Can you work these out from the model? Positions are in its coordinate system, mm. A direction names the side the tool comes from. Coordinates: 2 decimals unless noted, no trailing zeros. Order: outer loops, then holes, each group sorted by start corner. A loop starts at its lowest first (then second) coordinate and runs counter-clockwise, first axis right, second up. Notation, with made-up numbers: (63, -20.75) -> (107, -20.75) arc R16 ccw to (107, 7.25) -> close; hole circle Ø1 at (46.5, -27). An arc over 180 degrees is marked (long way). Answer in a Markdown table with one row per item.
```python
from build123d import *

# Parameters (mm, degrees)
SKETCH1_R           = 2
SKETCH1_W           = 52
SKETCH1_H           = 17
BOSS_EXTRUDE1_DEPTH = 3
BOSS_EXTRUDE2_DEPTH = 1
BOSS_EXTRUDE3_DEPTH = 2


with BuildPart() as part:
    # Sketch1 → Boss-Extrude1 (new body)
    with BuildSketch(Plane.XY):
        with BuildLine():
            Line((-44.9909991, 29.1), (44.9909991, 29.1))
            ThreePointArc((44.9909991, 29.1), (0, -15), (-44.9909991, 29.1))
        make_face()
        with Locations((-33, 11.5)):
            Circle(SKETCH1_R, mode=Mode.SUBTRACT)
        with Locations((33, 11.5)):
            Circle(SKETCH1_R, mode=Mode.SUBTRACT)
        with Locations((0, 11.5)):
            Rectangle(SKETCH1_W, SKETCH1_H, mode=Mode.SUBTRACT)
    extrude(amount=BOSS_EXTRUDE1_DEPTH)

    # Sketch4 → Boss-Extrude2 (add)
    with BuildSketch(Plane(origin=(0, 28.1, 0), x_dir=(1, 0, 0), z_dir=(0, 1, 0))):
        with BuildLine():
            Line((-25.4, 42.912140351), (-44.9909991, 0))
            Line((-44.9909991, 0), (44.9909991, 0))
            Line((44.9909991, 0), (25.4, 42.912140351))
            ThreePointArc((25.4, 42.912140351), (0, 33), (-25.4, 42.912140351))
        make_face()
    extrude(amount=BOSS_EXTRUDE2_DEPTH)

    # Sketch5 → Boss-Extrude3 (add)
    with BuildSketch(Plane(origin=(0, 29.1, 0), x_dir=(1, 0, 0), z_dir=(0, 1, 0))):
        with BuildLine():
            Line((-37.365311148, 16.703313087), (-44.9909991, 0))
            Line((-44.9909991, 0), (-44.9909991, -3))
            Line((-44.9909991, -3), (44.9909991, -3))
            Line((44.9909991, -3), (44.9909991, 0))
            Line((44.9909991, 0), (37.365311148, 16.703313087))
            ThreePointArc((37.365311148, 16.703313087), (0, 5), (-37.365311148, 16.703313087))
        make_face()
    extrude(amount=BOSS_EXTRUDE3_DEPTH)


solid = part.part
```
(1) Will these pins go through, and if not, where does the flat tip stop? pin 1 Ø13 at (x, y) = (11, -3.5) entering from -Z; pin 2 Ø8 at (x, z) = (35, -18.5) entering from -Y; pin 3 Ø6 at (x, z) = (-29.5, -36) entering from +Y.
Response values:
| item | result |
|---|---|
| pin 1 | z = 0 |
| pin 2 | y = 28.1 |
| pin 3 | y = 29.1 |
(2) On a 3-axis mill with a long thin cutter (end or side, diameter ignored), from which of +Z, -Z, +X, -X, +Y, -Y can I reach the whole of each face in a straight line? I mean faces 4 (the flat face through (-1, 29.1, -20)), 5 (the flat face through (-1, 28.1, -17)), 6 (the flat face through (26, 11, 1)). Say none if no direction works.
Response values:
| item | result |
|---|---|
| face 4 | -Z, +Y |
| face 5 | -Z, +X, -X, -Y |
| face 6 | +Z, -Z |
(3) Suppose I cut it at A-A (x = 0). Please give me the cut outline in (y, z), and give its area (3 significant figures).
Response values:
| item | result |
|---|---|
| outline | (-15, 0) -> (3, 0) -> (3, 3) -> (-15, 3) -> close; (20, 0) -> (28.1, 0) -> (28.1, -33) -> (29.1, -33) -> (29.1, -5) -> (31.1, -5) -> (31.1, 3) -> (20, 3) -> close |
| area | 130 mm2 |
(4) Suppose I cut it at B-B (y = 11.5). Please give me the cut outline in (x, z).
Response values:
| item | result |
|---|---|
| outline | (-41.02, 0) -> (-35, 0) -> (-35, 3) -> (-41.02, 3) -> close; (-31, 0) -> (-26, 0) -> (-26, 3) -> (-31, 3) -> close; (26, 0) -> (31, 0) -> (31, 3) -> (26, 3) -> close; (35, 0) -> (41.02, 0) -> (41.02, 3) -> (35, 3) -> close |
(5) Suppose I cut it at C-C (y = 30). Please give me the cut outline in (x, z).
Response values:
| item | result |
|---|---|
| outline | (-44.99, 0) -> (-37.37, -16.7) arc R65.5 cw to (37.37, -16.7) -> (44.99, 0) -> (44.99, 3) -> (-44.99, 3) -> close |
(6) I need wall thicknesses on line 1 (X direction, y = 11, z = 1); line 2 (Y direction, x = 33, z = 2.15); line 3 (Z direction, x = -36, y = 3.5). Which ranges of each line are inside material? Lowest first, please. Write a range as [from, to].
Response values:
| item | result |
|---|---|
| line 1 | [-40.79, -34.94], [-31.06, -26], [26, 31.06], [34.94, 40.79] |
| line 2 | [-0.59, 9.5], [13.5, 31.1] |
| line 3 | [0, 3] |
(7) We'd pull the mould along X, two halves only. Please class faces 1 (the flat face through (1, 2, 0)), 2 (the flat face through (44.991, 30, 2)), 3 (the flat face through (0, 20, 1)): +X half, -X half, draft (parallel to the pull), parting line (faces both ways), or undercut.
Response values:
| item | result |
|---|---|
| face 1 | draft |
| face 2 | +X half |
| face 3 | undercut |
(8) Suppose I cut it at D-D (z = -8). Please give me the cut outline in (x, y).
Response values:
| item | result |
|---|---|
| outline | (-41.34, 28.1) -> (41.34, 28.1) -> (41.34, 31.1) -> (19.6, 31.1) -> (19.6, 29.1) -> (-19.6, 29.1) -> (-19.6, 31.1) -> (-41.34, 31.1) -> close |
